Check sheet for the modelled part. Datum: model origin and axes. Units: mm. Round coordinates to 2 decimals unless told otherwise and drop trailing zeros. Loops run counter-clockwise (first coordinate to the right, second up) from the corner with the lowest first, then second, coordinate; pieces in that order, holes last. Notation, with made-up numbers: (-40, 80.25) - (-22, 80.25) arc R21 cw to (-22, 98.25) - close; hole circle Ø1 at (86.5, -11). An arc over 180 degrees is marked (long way). Answer in a Markdown table with one row per item. Add a question column.
(1) Gauge pin test, flat end, axial feed: pin 1 (6 mm diameter, centred on x = -25, y = -9.21, fed in from -Z). Record the tip position at first contact, or that the pin passes through.
(2) Cross-section at B-B on x = 25. Enter the section's corners in (y, z), then the cut area to 3 significant figures.
(3) Thickness scan on line 1 along Y through (x, z) = (25, 3); line 2 along X through (y, z) = (-9, 7); line 3 along X through (y, z) = (-8, 7.5). Record the ranges inside material, lowest first.
(4) Cross-section at A-A on y = 3. Enter the section's corners in (x, z).
(5) Cross-section at C-C on z = 5.75. Enter the section's corners in (x, y).
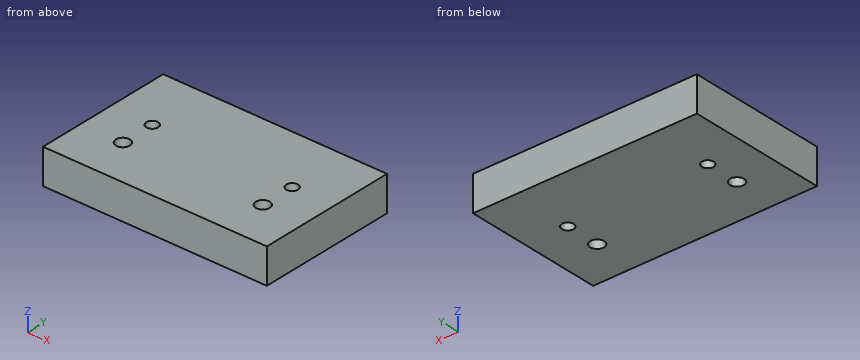
from build123d import *

# Parameters (mm, degrees)
SKETCH1_W             = 80
SKETCH1_H             = 50
EXTRUDE1_DEPTH        = 12.5
M6_TAPPED_HOLE1_D     = 5
M5_TAPPED_HOLE1_D     = 4.2
M5_TAPPED_HOLE1_DEPTH = 12.5


with BuildPart() as part:
    # Sketch1 → Extrude1 (new body)
    with BuildSketch(Plane.XY):
        Rectangle(SKETCH1_W, SKETCH1_H)
    extrude(amount=EXTRUDE1_DEPTH)

    # M6 Tapped Hole1 (through all)
    with Locations(Plane.XY.offset(12.5)):
        with Locations((-25, -9.206258577), (25, -9.206258577)):
            Hole(M6_TAPPED_HOLE1_D / 2)

    # M5 Tapped Hole1
    with Locations(Plane.XY.offset(12.5)):
        with Locations((-25, 3), (25, 3)):
            Hole(M5_TAPPED_HOLE1_D / 2, depth=M5_TAPPED_HOLE1_DEPTH)


solid = part.part
Answers:
| question | item | result |
|---|---|---|
| 1 | pin 1 | stops at z = 0 |
| 2 | outline | (-25, 0) - (-11.71, 0) - (-11.71, 12.5) - (-25, 12.5) - close; (-6.71, 0) - (0.9, 0) - (0.9, 12.5) - (-6.71, 12.5) - close; (5.1, 0) - (25, 0) - (25, 12.5) - (5.1, 12.5) - close |
| 2 | area | 510 mm^2 |
| 3 | line 1 | y = -25 to -11.71, -6.71 to 0.9, 5.1 to 25 |
| 3 | line 2 | x = -40 to -27.49, -22.51 to 22.51, 27.49 to 40 |
| 3 | line 3 | x = -40 to -27.19, -22.81 to 22.81, 27.19 to 40 |
| 4 | outline | (-40, 0) - (-27.1, 0) - (-27.1, 12.5) - (-40, 12.5) - close; (-22.9, 0) - (22.9, 0) - (22.9, 12.5) - (-22.9, 12.5) - close; (27.1, 0) - (40, 0) - (40, 12.5) - (27.1, 12.5) - close |
| 5 | outline | (-40, -25) - (40, -25) - (40, 25) - (-40, 25) - close; hole circle Ø5 at (-25, -9.21); hole circle Ø4.2 at (-25, 3); hole circle Ø5 at (25, -9.21); hole circle Ø4.2 at (25, 3) |
